Here's how the part is built. I have some questions about the finished solid (model axes, mm). A direction names the side the tool comes from. Give positions to 0.01 mm unless a question says otherwise; leave off trailing zeros. Loops run counter-clockwise (first coordinate to the right, second up) from the corner with the lowest first, then second, coordinate; pieces in that order, holes last.
Q1. Suppose I cut it at A-A (z = 13.25). List the corners of the cut face in (x, y) for me.
Q2. Suppose I cut it at C-C (y = -16.5). List the corners of the cut face in (x, z) for me, and give its area (3 significant figures).
Q3. For faces 4 (the face through (-80, 0, 8)), 5 (the face through (29, 9, 9)), which set-ups out of +Z, -Z, +X, -X, +Y, -Y let a thin tool reach every point of the face, with its end or its side?
Q4. Suppose I cut it at B-B (x = -70). List the corners of the cut face in (y, z) for me.
Q5. Suppose I cut it at D-D (x = 189). List the corners of the cut face in (y, z) for me.
Q6. I need wall thicknesses on probe 1 along Y at (x, z) = (37.25, 11.75); probe 2 along Y at (x, z) = (-70, 12.75); probe 3 along Y at (x, z) = (-186, 6). Which ranges of each line are inside material? Lowest first, please.
Q7. I'm going to push flat-ended pins straight in: P1, Ø10.5, axis at x = 0, y = 37.25, coming from the -Z side; P2, Ø2, axis at x = 122.5, y = -181, coming from the -Z side; P3, Ø8, axis at x = -151, z = 6, coming from the -Y side; P4, Ø6, axis at y = -57, z = 1.5, coming from the -X side. Where does each tip first touch, or does it pass through?
Q8. Thinking about a two-plate mould opening in X: for faces 1 (the face through (-222.198, -170.376, 7.888)), 2 (the face through (58, 4, 16)), 3 (the face through (-9.59, 43.2, 4.44)), which applies, pulls with the +X half, pulls with the -X half, needs draft (parallel to the pull), parting line crosses it, or undercut?
```python
from build123d import *

# Parameters (mm, degrees)
F0_R     = 280
F1_DEPTH = 16
F2_R     = 30
F2_R_2   = 10
F2_R_3   = 4.5
F3_DEPTH = 25
F4_R     = 44.25
F5_DEPTH = 9


with BuildPart() as f1:
    # F0 (on Top) → F1 (new body)
    with BuildSketch(Plane.XY):
        Circle(F0_R)
    extrude(amount=F1_DEPTH)

    # F2 (on face) → F3 (cut)
    with BuildSketch(Plane.XY.offset(16)):
        Circle(F2_R)
        with Locations((-70, 0)):
            Circle(F2_R_2)
        with Locations((-37.25, 0)):
            Circle(F2_R_3)
        with Locations((0, 37.25)):
            Circle(F2_R_3)
        with Locations((37.25, 0)):
            Circle(F2_R_3)
        with Locations((0, -37.25)):
            Circle(F2_R_3)
    extrude(amount=-F3_DEPTH, mode=Mode.SUBTRACT)

    # F4 (on face) → F5 (cut)
    with BuildSketch(Plane(origin=(0, 0, 0), x_dir=(1, 0, 0), z_dir=(0, 0, -1))):
        Circle(F4_R)
    extrude(amount=-F5_DEPTH, mode=Mode.SUBTRACT)


solid = f1.part
```
Solutions:
1. outline: circle Ø560 at (0, 0); hole circle Ø20 at (-70, 0); hole circle Ø9 at (-37.25, 0); hole circle Ø60 at (0, 0); hole circle Ø9 at (0, -37.25); hole circle Ø9 at (0, 37.25); hole circle Ø9 at (37.25, 0)
2. outline: (-279.51, 0) - (-41.06, 0) - (-41.06, 9) - (-25.05, 9) - (-25.05, 16) - (-279.51, 16) - close; (25.05, 9) - (41.06, 9) - (41.06, 0) - (279.51, 0) - (279.51, 16) - (25.05, 16) - close
2. area: 7,850 mm2
3. face 4: +Z, -Z
3. face 5: -Z
4. outline: (-271.11, 0) - (-10, 0) - (-10, 16) - (-271.11, 16) - close; (10, 0) - (271.11, 0) - (271.11, 16) - (10, 16) - close
5. outline: (-206.59, 0) - (206.59, 0) - (206.59, 16) - (-206.59, 16) - close
6. probe 1: y = -277.51 to -4.5, 4.5 to 277.51
6. probe 2: y = -271.11 to -10, 10 to 271.11
6. probe 3: y = -209.29 to 209.29
7. P1: stops at z = 9
7. P2: stops at z = 0
7. P3: stops at y = -238.31
7. P4: stops at x = -274.74
8. face 1: parting line crosses it
8. face 2: needs draft
8. face 3: undercut
